Source: CAD feature listing. Evaluate the final solid. Frame: model axes, mm. A direction names the side the tool comes from. Coordinates: 2 decimals unless noted, no trailing zeros. Order: outer loops, then holes, each group sorted by start corner. A loop starts at its lowest first (then second) coordinate and runs counter-clockwise, first axis right, second up.
Item 1: Contact query for flat-ended pins moving along their axis: P1, Ø1.5, axis at x = -1.5, z = -0.5, coming from the -Y side; P2, Ø3, axis at x = 6.5, z = -3, coming from the +Y side (3 decimals); P3, Ø1.1, axis at x = -1.5, z = 0, coming from the +Y side; P4, Ø1.9, axis at y = 0.5, z = -0.5, coming from the -X side. Output: stop coordinate, or through.
Item 2: Reachability of faces 1 (the flat face through (12.7, 0, 0)), 2 (the flat face through (-1.232, -0.587, 1.036)), 3 (the flat face through (0, 2, -2)) from +Z, -Z, +X, -X, +Y, -Y: full face, straight path, thin tool, end or side. Return the list, or none.
Item 3: Ray query, line 1 (Z direction, x = 7.5, y = -0.75); line 2 (X direction, y = 1, z = -0.5); line 3 (Y direction, x = -0.5, z = 2.25). Return the intervals inside material, ascending.
Item 4: Section A-A on x = 3.75. Return the cut outline in (y, z).
Item 5: Mould query, pull axis Y, two halves, no side actions, for faces 4 (the flat face through (-2.21, 1, -1)), 5 (the flat face through (-1, 1.191, 0)), 6 (the cylindrical face through (6.199, 1.987, 0.626)). Classes: released by +Y, released by -Y, zero draft, split by the parting line, or undercut.
Autodesk Inventor part; units mm, degrees
ref_plane "screw_XY" through (0, 0, 0) normal (1, 0, 0) x (0, 0, -1)
ref_plane "screw_YZ" through (0, 0, 0) normal (0, 0, -1) x (0, 1, 0)
ref_plane "screw_ZX" through (0, 0, 0) normal (0, 1, 0) x (1, 0, 0)
sketch "Sketch_1" plane through (0, 0, 0) normal (0, 0, 1) x (1, 0, 0)
  line L0 (12.7, 0) -> (-2.2098, 0)
  line L1 (-2.2098, 0) -> (-2.2098, 2.0828)
  arc A0 (-0.2794, 3.9688) -> (-2.2098, 2.0828) centre (1.7151, -0.0037) ccw
  line L2 (-0.2794, 3.9688) -> (0, 3.9688)
  line L3 (0, 3.9688) -> (0, 2.0828)
  line L4 (0, 2.0828) -> (12.2276, 2.0828)
  line L5 (12.2276, 2.0828) -> (12.7, 1.6104)
  line L6 (12.7, 1.6104) -> (12.7, 0)
  line L7 (12.7, 0) -> (-2.2098, 0)
revolve "Revolution1" add sketch "Sketch_1" angle 360 about axis through (12.7, 0, 0) along (1, 0, 0)
thread "Thread1"
sketch "Sketch_3" plane through (-2.2098, 0, 0) normal (1, 0, 0) x (0, 0, -1)
  line L0 (-1.3748, 0) -> (-0.6874, -1.1906)
  line L1 (-0.6874, -1.1906) -> (0.6874, -1.1906)
  line L2 (0.6874, -1.1906) -> (1.3748, 0)
  line L3 (1.3748, 0) -> (0.6874, 1.1906)
  line L4 (0.6874, 1.1906) -> (-0.6874, 1.1906)
  line L5 (-0.6874, 1.1906) -> (-1.3748, 0)
extrude "Extrusion1" cut sketch "Sketch_3" along normal mid plane 3.9675
ref_plane "screw_XY" through (0, 0, 0) normal (1, 0, 0) x (0, 0, -1)
ref_plane "screw_YZ" through (0, 0, 0) normal (0, 0, -1) x (0, 1, 0)
ref_plane "screw_ZX" through (0, 0, 0) normal (0, 1, 0) x (1, 0, 0)
ref_plane "to_nut_XY" through (12.7, 0, 0) normal (1, 0, 0) x (0, 0, -1)
ref_plane "to_nut_YZ" through (12.7, 0, 0) normal (0, 0, -1) x (0, 1, 0)
ref_plane "to_nut_ZX" through (12.7, 0, 0) normal (0, 1, 0) x (1, 0, 0)
properties part number "3024"
Answer list:
1. P1: stops at y = -3.67
1. P2: stops at y = 1.445
1. P3: stops at y = 3.55
1. P4: stops at x = -2.21
2. face 1: +Z, -Z, +X, +Y, -Y
2. face 2: -X
2. face 3: +X
3. line 1: z = -1.94 to 1.94
3. line 2: x = -0.23 to 12.7
3. line 3: y = -3.12 to 3.12
4. outline: circle Ø4.17 at (0, 0)
5. face 4: zero draft
5. face 5: undercut
5. face 6: split by the parting line
